from build123d import *

# Parameters (mm, degrees)
F0_R     = 10
F1_DEPTH = 40
F2_R     = 8
F3_DEPTH = 35
F5_DEPTH = 2


with BuildPart() as f1:
    # F0 (on Top) → F1 (new body)
    with BuildSketch(Plane.XY):
        Circle(F0_R)
    extrude(amount=F1_DEPTH)

    # F2 (on face) → F3 (cut)
    with BuildSketch(Plane.XY.offset(40)):
        Circle(F2_R)
    extrude(amount=-F3_DEPTH, mode=Mode.SUBTRACT)

    # F4 (on face) → F5 (join)
    with BuildSketch(Plane(origin=(0, 0, 0), x_dir=(1, 0, 0), z_dir=(0, 0, -1))):
        with BuildLine():
            Line((-10, 0), (0, 0))
            Line((0, 0), (10, 0))
            ThreePointArc((10, 0), (0, 10), (-10, 0))
        make_face()
        with BuildLine():
            Line((10, 0), (0, 0))
            Line((0, 0), (-10, 0))
            ThreePointArc((-10, 0), (0, -10), (10, 0))
        make_face()
        with BuildLine():
            ThreePointArc((-10, 0), (0, 10), (10, 0))
            ThreePointArc((10, 0), (7.4121106103, 13.8021737418), (0, 25.7293606605))
            Line((0, 25.7293606605), (-14.750656168, 12.223134592))
            ThreePointArc((-14.750656168, 12.223134592), (-11.2294172691, 6.5569381818), (-10, 0))
        make_face()
        with BuildLine():
            ThreePointArc((0, -25.7293606605), (7.4121106103, -13.8021737418), (10, 0))
            ThreePointArc((10, 0), (0, -10), (-10, 0))
            ThreePointArc((-10, 0), (-11.2294172691, -6.5569381818), (-14.750656168, -12.223134592))
            Line((-14.750656168, -12.223134592), (0, -25.7293606605))
        make_face()
    extrude(amount=F5_DEPTH)


solid = f1.part
Design review of the part built by this model. Coordinates are the model's own, in mm. A direction names the side the tool comes from. Give positions to 0.01 mm unless a question says otherwise; leave off trailing zeros. Loops run counter-clockwise (first coordinate to the right, second up) from the corner with the lowest first, then second, coordinate; pieces in that order, holes last. Notation, with made-up numbers: (-38.75, 61.5) - (-31.75, 61.5) arc R26 cw to (-31.75, 95.5) - close; hole circle Ø2 at (-6.5, -31). An arc over 180 degrees is marked (long way). Write item = value, one per line.
1) Take a section at C-C on y = -3. State the section outline as (x, z) points, and give its area (3 significant figures).
Result sheet:
outline = (-10.25, -2) - (9.88, -2) - (9.88, 0) - (9.54, 0) - (9.54, 40) - (7.42, 40) - (7.42, 5) - (-7.42, 5) - (-7.42, 40) - (-9.54, 40) - (-9.54, 0) - (-10.25, 0) - close
area = 284 mm2
2) To check wall thickness, follow line 1 (Y direction, x = 0, z = 15.5); line 2 (Z direction, x = -4.5, y = -3); line 3 (X direction, y = -1, z = 20). State the ranges of each line that lie inside material, in increasing order.
Result sheet:
line_1 = -10 to -8, 8 to 10
line_2 = -2 to 5
line_3 = -9.95 to -7.94, 7.94 to 9.95
3) Draft analysis for pull direction Y (two halves, no side actions). For faces 1 (the face through (-2.17, -9.76, 19.72)), 2 (the face through (-3, 13, 0)), 3 (the face through (-7.27, -19.07, -0.99)), 4 (the face through (-1.73, -7.81, 22.74)), state which applies: +Y half, -Y half, draft (parallel to the pull), parting line (faces both ways), or undercut.
Result sheet:
face_1 = parting line
face_2 = draft
face_3 = -Y half
face_4 = undercut
4) Clearance check with flat-ended pins moving along their axes: pin 1 Ø6 at (y, z) = (-3.5, 32) entering from -X; pin 2 Ø4 at (y, z) = (-4, 8.5) entering from +X; pin 3 Ø12 at (x, z) = (-4.5, 11.5) entering from +Y; pin 4 Ø8 at (x, y) = (3.5, -4) entering from +Z. State where each tip first meets the part, or that it passes through.
Result sheet:
pin_1 = -9.99
pin_2 = 9.8
pin_3 = 10
pin_4 = 40
5) Take a section at A-A on z = 6. State the section outline as (x, y) points.
Result sheet:
outline = circle Ø20 at (0, 0); hole circle Ø16 at (0, 0)
6) Take a section at D-D on y = 21. State the section outline as (x, z) points.
Result sheet:
outline = (-5.17, -2) - (3.69, -2) - (3.69, 0) - (-5.17, 0) - close
7) Take a section at B-B on x = 2. State the section outline as (y, z) points.
Result sheet:
outline = (-23.36, -2) - (23.36, -2) - (23.36, 0) - (9.8, 0) - (9.8, 40) - (7.75, 40) - (7.75, 5) - (-7.75, 5) - (-7.75, 40) - (-9.8, 40) - (-9.8, 0) - (-23.36, 0) - close
8) Tool access review of faces 5 (the face through (0, 8.2, 40)), 6 (the face through (0, 0, 5)): name each direction out of +Z, -Z, +X, -X, +Y, -Y from which nothing blocks a thin tool from reaching the whole face with its end or side.
Result sheet:
face_5 = +Z, +X, -X, +Y, -Y
face_6 = +Z
